from build123d import *

# Parameters (mm, degrees)
F1_R     = 3.15
F2_DEPTH = 4
F3_DEPTH = 23
F4_DEPTH = 19
F5_R     = 5
F6_SIZE  = 5


# Not quite as in the source:
# - a feature names something its author has since deleted; it is built from what else it names


with BuildPart() as f2:
    # F1 (on Top) → F2 (new body)
    with BuildSketch(Plane.XY):
        Polygon((-4.4541987248, 17.7165100388), (-10.2041987248, 17.7165100388), (-10.2041987248, 13.7165100388), (-6.2041987248, 13.7165100388), (-4.4541987248, 13.7165100388), align=None)
        Polygon((-6.2041987248, 13.7165100388), (-10.2041987248, 13.7165100388), (-10.2041987248, -11.5894424588), (15.2958012752, -11.5894424588), (15.2958012752, 13.7165100388), (11.2958012752, 13.7165100388), (11.2958012752, -3.2953930364), (-6.2041987248, -3.2834899612), align=None)
        with Locations((2.5458012752, -7.4394424588)):
            Circle(F1_R, mode=Mode.SUBTRACT)
        Polygon((9.5458012752, 17.7165100388), (-4.4541987248, 17.7165100388), (-4.4541987248, 13.7165100388), (-3.9542341456, 13.7165100388), (9.5458012752, 13.7165100388), align=None)
        Polygon((15.2958012752, 17.7165100388), (9.5458012752, 17.7165100388), (9.5458012752, 13.7165100388), (11.2958012752, 13.7165100388), (15.2958012752, 13.7165100388), align=None)
    extrude(amount=F2_DEPTH)

    # F1 (on Top) → F3 (join)
    with BuildSketch(Plane.XY):
        Polygon((-4.4541987248, 17.7165100388), (-10.2041987248, 17.7165100388), (-10.2041987248, 13.7165100388), (-6.2041987248, 13.7165100388), (-4.4541987248, 13.7165100388), align=None)
        Polygon((9.5458012752, 17.7165100388), (-4.4541987248, 17.7165100388), (-4.4541987248, 13.7165100388), (-3.9542341456, 13.7165100388), (9.5458012752, 13.7165100388), align=None)
        Polygon((15.2958012752, 17.7165100388), (9.5458012752, 17.7165100388), (9.5458012752, 13.7165100388), (11.2958012752, 13.7165100388), (15.2958012752, 13.7165100388), align=None)
    extrude(amount=F3_DEPTH)

    # F1 (on Top) → F4 (cut)
    with BuildSketch(Plane.XY):
        Polygon((9.5458012752, 17.7165100388), (-4.4541987248, 17.7165100388), (-4.4541987248, 13.7165100388), (-3.9542341456, 13.7165100388), (9.5458012752, 13.7165100388), align=None)
    extrude(amount=F4_DEPTH, mode=Mode.SUBTRACT)

    # F5
    f5_edges = [f2.edges().sort_by_distance(p)[0] for p in [
        (-10.204199, -11.589442, 2),
        (15.295801, -11.589442, 2),
        (15.295801, 15.71651, 23),
        (-10.204199, 15.71651, 23),
    ]]
    fillet(f5_edges, radius=F5_R)

    # F6
    f6_edges = [f2.edges().sort_by_distance(p)[0] for p in [
        (-8.204199, 13.71651, 4),
        (13.295801, 13.71651, 4),
    ]]
    chamfer(f6_edges, length=F6_SIZE)


solid = f2.part
Geometry: final body of the model. Coordinates: model frame, mm. A direction names the side the tool comes from. Round coordinates to 2 decimals unless told otherwise and drop trailing zeros. Write each loop counter-clockwise with the first axis right and the second up, starting at its lowest first coordinate (ties: lowest second). Pieces come first, ordered by that corner, then holes. Notation, with made-up numbers: M 22,74 L 57,74 A11 cw 57,90 Z; hole C 56.25,16.25 d5. An arc over 180 degrees is marked long. Write item = value, one per line.
Item 1: Pin query (flat end, axial travel): P1, Ø4, axis at x = 2.55, y = -7.44, coming from the +Z side; P2, Ø2, axis at x = 5, y = 16.5, coming from the -Z side; P3, Ø10, axis at x = 6.5, y = -6, coming from the +Z side; P4, Ø1, axis at x = -4, z = 12.5, coming from the -Y side. Return the tip coordinate at first contact, or that it passes through.
Findings:
P1 = through
P2 = 19
P3 = 4
P4 = 13.72
Item 2: Material intervals for line 1 along X through (y, z) = (2.25, 2.25); line 2 along Z through (x, y) = (-8.5, -6); line 3 along Y through (x, z) = (-6.75, 13), sorted ascending. Write a range as [from, to].
Findings:
line_1 = [-10.2, -6.2], [11.3, 15.3]
line_2 = [0, 4]
line_3 = [13.72, 17.72]
Item 3: Section query B-B on y = 8.25. Return loops of the section in (x, z).
Findings:
outline = M -10.2,0 L -6.2,0 L -6.2,4 L -10.2,4 Z; M 11.3,0 L 15.3,0 L 15.3,4 L 11.3,4 Z
Item 4: Pull-direction query (X, two-part tool) for faces 1 (the face through (-4.454, 16, 9)), 2 (the face through (-8.778, 15.689, 21.496)), 3 (the face through (-3, -6, 0)); classes: pulls with the +X half, pulls with the -X half, needs draft (parallel to the pull), parting line crosses it, or undercut.
Findings:
face_1 = undercut
face_2 = pulls with the -X half
face_3 = needs draft
Item 5: Access query for faces 4 (the face through (-10.204, 11, 5)), 5 (the face through (9.546, 16, 9)), 6 (the face through (2, 16, 19)), 7 (the face through (11.296, 7, 2)). Directions: +Z, -Z, +X, -X, +Y, -Y. A direction counts if a zero-diameter tool reaches every point of the face in a straight line with its end or side. Return the directions, or none.
Findings:
face_4 = +Z, -Z, -X, +Y, -Y
face_5 = -Z, +Y
face_6 = -Z, +Y, -Y
face_7 = +Z, -Z
Item 6: Section query D-D on y = 14.75. Return loops of the section in (x, z).
Findings:
outline = M -10.2,0 L -4.45,0 L -4.45,19 L 9.55,19 L 9.55,0 L 15.3,0 L 15.3,18 A5 ccw 10.3,23 L -5.2,23 A5 ccw -10.2,18 Z
Item 7: Section query A-A on z = 12.75. Return loops of the section in (x, y), then the cut area to 3 significant figures.
Findings:
outline = M -10.2,13.72 L -4.45,13.72 L -4.45,17.72 L -10.2,17.72 Z; M 9.55,13.72 L 15.3,13.72 L 15.3,17.72 L 9.55,17.72 Z
area = 46.0 mm^2
Item 8: Section query C-C on x = 4. Return loops of the section in (y, z).
Findings:
outline = M -11.59,0 L -10.23,0 L -10.23,4 L -11.59,4 Z; M -4.65,0 L -3.29,0 L -3.29,4 L -4.65,4 Z; M 13.72,19 L 17.72,19 L 17.72,23 L 13.72,23 Z
